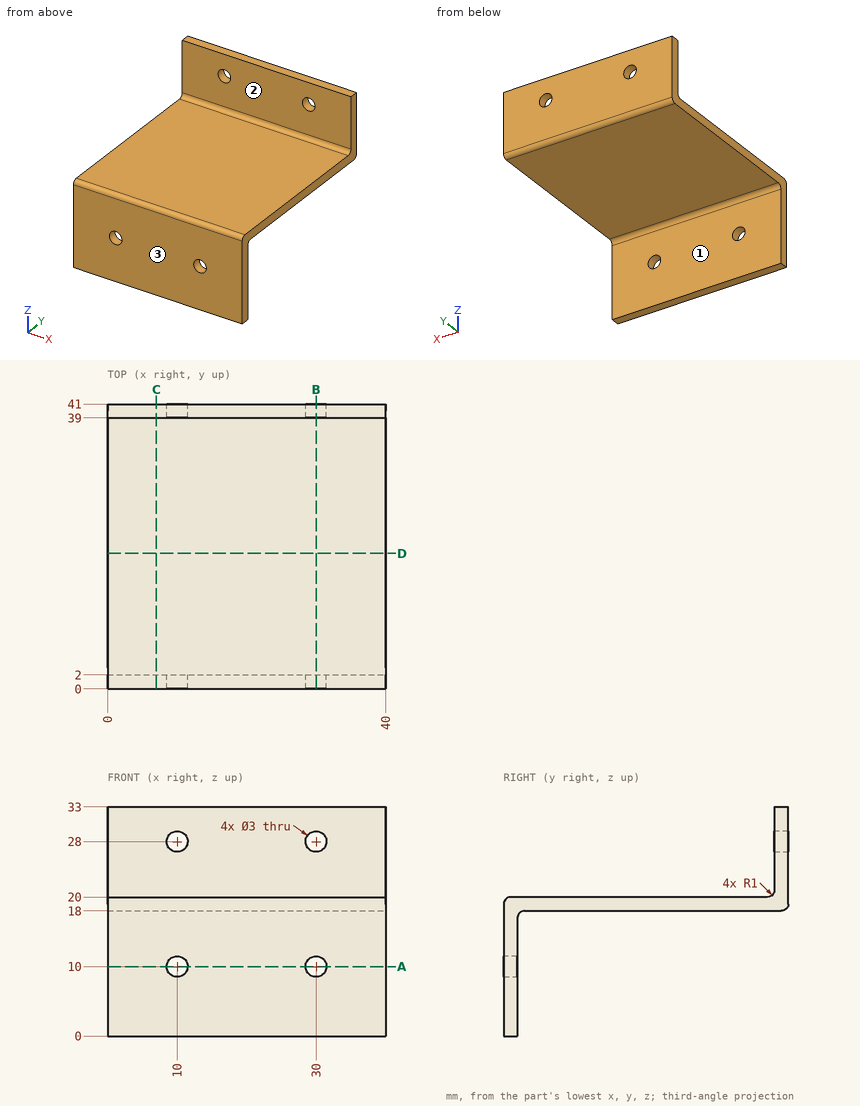
Could you check a few things on this drawing? It's one solid part, dimensions in mm from its lowest x, y, z. A direction names the side the tool comes from. Give positions to 0.01 mm unless a question says otherwise; leave off trailing zeros. Write each loop counter-clockwise with the first axis right and the second up, starting at its lowest first coordinate (ties: lowest second). Pieces come first, ordered by that corner, then holes. Notation, with made-up numbers: (83.5, 36) -> (126.5, 36) arc R30 cw to (126.5, 68) -> close; hole circle Ø11 at (-11, -28). An arc over 180 degrees is marked (long way). Write each question's results on one line, items separated by ' | '.
1. I want a section at C-C, the plane x = 7. Write out the boundary of the cut face in (y, z), then the cut area to 3 significant figures.
Check sheet entries:
outline: (0, 0) -> (2, 0) -> (2, 17) arc R1 cw to (3, 18) -> (40, 18) arc R1 ccw to (41, 19) -> (41, 33) -> (39, 33) -> (39, 21) arc R1 cw to (38, 20) -> (1, 20) arc R1 ccw to (0, 19) -> close | area: 144 mm²
2. I want a section at A-A, the plane z = 10. Write out the boundary of the cut face in (x, y).
Check sheet entries:
outline: (0, 0) -> (8.5, 0) -> (8.5, 2) -> (0, 2) -> close; (11.5, 0) -> (28.5, 0) -> (28.5, 2) -> (11.5, 2) -> close; (31.5, 0) -> (40, 0) -> (40, 2) -> (31.5, 2) -> close
3. On a 3-axis mill with a long thin cutter (end or side, diameter ignored), from which of +Z, -Z, +X, -X, +Y, -Y can I reach the whole of each face in a straight line? I mean the marked faces 1, 2 and 3. Say none if no direction works.
Check sheet entries:
face 1: -Z, +X, -X, +Y | face 2: +Z, +X, -X, -Y | face 3: +Z, -Z, +X, -X, -Y
4. Will these pins go through, and if not, where does the flat tip stop? pin 1 Ø4 at (x, y) = (25.5, 32) entering from +Z; pin 2 Ø8 at (x, y) = (10, 20) entering from -Z; pin 3 Ø4 at (x, z) = (30, 10) entering from +Y.
Check sheet entries:
pin 1: stops at z = 20 | pin 2: stops at z = 18 | pin 3: stops at y = 2
5. I want a section at B-B, the plane x = 30. Write out the boundary of the cut face in (y, z).
Check sheet entries:
outline: (0, 0) -> (2, 0) -> (2, 8.5) -> (0, 8.5) -> close; (0, 11.5) -> (2, 11.5) -> (2, 17) arc R1 cw to (3, 18) -> (40, 18) arc R1 ccw to (41, 19) -> (41, 26.5) -> (39, 26.5) -> (39, 21) arc R1 cw to (38, 20) -> (1, 20) arc R1 ccw to (0, 19) -> close; (39, 29.5) -> (41, 29.5) -> (41, 33) -> (39, 33) -> close
6. I want a section at D-D, the plane y = 19.5. Write out the boundary of the cut face in (x, z), then the cut area to 3 significant figures.
Check sheet entries:
outline: (0, 18) -> (40, 18) -> (40, 20) -> (0, 20) -> close | area: 80.0 mm²
7. I need wall thicknesses on L1, parallel to X at y = 1.65, z = 10; L2, parallel to Z at x = 23, y = 29; L3, parallel to Y at x = 21, z = 8.5. Which ranges of each line are inside material? Lowest first, please.
Check sheet entries:
L1: x = 0 to 8.5, 11.5 to 28.5, 31.5 to 40 | L2: z = 18 to 20 | L3: y = 0 to 2
